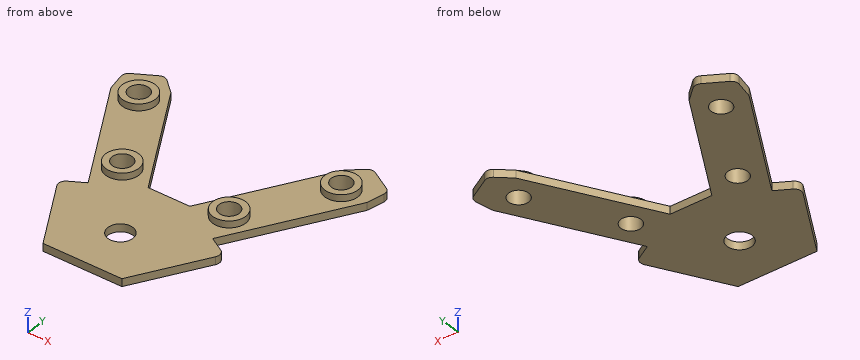
```python
from build123d import *

# Parameters (mm, degrees)
SKETCH1_R             = 2.6
BOSS_EXTRUDE1_DEPTH   = 1.6
SKETCH2_R             = 3.45
BOSS_EXTRUDE2_DEPTH   = 1.4
M5X0_8_TAPPED_HOLE1_D = 4.2


with BuildPart() as part:
    # Sketch1 → Boss-Extrude1 (new body)
    with BuildSketch(Plane.XY):
        with BuildLine():
            Line((-4.364768035, 13.06), (4.364768035, 13.06))
            Line((4.364768035, 13.06), (18.114768035, 36.875698604))
            Line((18.114768035, 36.875698604), (20.854894903, 39.305509792))
            ThreePointArc((20.854894903, 39.305509792), (21.698970531, 39.675572625), (22.600099833, 39.482243506))
            Line((22.600099833, 39.482243506), (26.789690275, 37.063382336))
            ThreePointArc((26.789690275, 37.063382336), (27.407682855, 36.379646028), (27.509236854, 35.463623675))
            Line((27.509236854, 35.463623675), (26.775022073, 31.875698604))
            Line((26.775022073, 31.875698604), (13.025022073, 8.06))
            Line((13.025022073, 8.06), (16.056110986, 6.31))
            ThreePointArc((16.056110986, 6.31), (16.754999726, 5.399190462), (16.605149092, 4.260961894))
            Line((16.605149092, 4.260961894), (8.250335347, -10.21))
            Line((8.250335347, -10.21), (-8.250335347, -10.21))
            Line((-8.250335347, -10.21), (-16.605149092, 4.260961894))
            ThreePointArc((-16.605149092, 4.260961894), (-16.754999726, 5.399190462), (-16.056110986, 6.31))
            Line((-16.056110986, 6.31), (-13.025022073, 8.06))
            Line((-13.025022073, 8.06), (-26.775022073, 31.875698604))
            Line((-26.775022073, 31.875698604), (-27.509236854, 35.463623675))
            ThreePointArc((-27.509236854, 35.463623675), (-27.407682855, 36.379646028), (-26.789690275, 37.063382336))
            Line((-26.789690275, 37.063382336), (-22.600099833, 39.482243506))
            ThreePointArc((-22.600099833, 39.482243506), (-21.698970531, 39.675572625), (-20.854894903, 39.305509792))
            Line((-20.854894903, 39.305509792), (-18.114768035, 36.875698604))
            Line((-18.114768035, 36.875698604), (-4.364768035, 13.06))
        make_face()
        Circle(SKETCH1_R, mode=Mode.SUBTRACT)
    extrude(amount=BOSS_EXTRUDE1_DEPTH)

    # Sketch2 → Boss-Extrude2 (add)
    with BuildSketch(Plane.XY.offset(1.6)):
        with Locations((21.178557159, 32.18233703)):
            Circle(SKETCH2_R)
        with Locations((11.178557159, 14.861828954)):
            Circle(SKETCH2_R)
        with Locations((-11.178557159, 14.861828954)):
            Circle(SKETCH2_R)
        with Locations((-21.178557159, 32.18233703)):
            Circle(SKETCH2_R)
    extrude(amount=BOSS_EXTRUDE2_DEPTH)

    # M5x0.8 Tapped Hole1 (through all)
    with Locations(Plane.XY.offset(3)):
        with Locations((21.178557159, 32.18233703), (11.178557159, 14.861828954), (-11.178557159, 14.861828954), (-21.178557159, 32.18233703)):
            Hole(M5X0_8_TAPPED_HOLE1_D / 2)


solid = part.part
```
Input: part model. Units: mm. Frame: model coordinates. Give positions to 0.01 mm unless a question says otherwise; leave off trailing zeros. Order: outer loops, then holes, each group sorted by start corner. A loop starts at its lowest first (then second) coordinate and runs counter-clockwise, first axis right, second up. Notation, with made-up numbers: M 25,29.25 L 50,29.25 A20 cw 50,67.25 Z; hole C -6.75,88 d10. An arc over 180 degrees is marked long. Return JSON: item names as keys, results as strings.
1) Section query D-D on x = 11. Output: boundary loops of the cut face in (y, z).
Taken from the geometry:
{"outline": "M -5.45,0 L 12.77,0 L 12.77,3 L 11.42,3 L 11.42,1.6 L -5.45,1.6 Z; M 16.95,0 L 24.55,0 L 24.55,1.6 L 18.31,1.6 L 18.31,3 L 16.95,3 Z"}
2) Contact query for flat-ended pins moving along their axis: pin 1 (5.5 mm diameter, centred on x = -11.18, y = 14.86, fed in from -Z); pin 2 (1.5 mm diameter, centred on y = 22, z = 1.5, fed in from -X); pin 3 (1.3 mm diameter, centred on x = -1, z = 0.5, fed in from +Y); pin 4 (1 mm diameter, centred on y = 32, z = 0.5, fed in from +X). Output: stop coordinate, or through.
Taken from the geometry:
{"pin 1": "stops at z = 0", "pin 2": "stops at x = -21.51", "pin 3": "stops at y = 13.06", "pin 4": "stops at x = 26.9"}
3) Section query B-B on y = 28. Output: boundary loops of the cut face in (x, z).
Taken from the geometry:
{"outline": "M -24.54,0 L -12.99,0 L -12.99,1.6 L -24.54,1.6 Z; M 12.99,0 L 24.54,0 L 24.54,1.6 L 12.99,1.6 Z"}
4) Section query A-A on x = 0. Output: boundary loops of the cut face in (y, z), and give its area (3 significant figures).
Taken from the geometry:
{"outline": "M -10.21,0 L -2.6,0 L -2.6,1.6 L -10.21,1.6 Z; M 2.6,0 L 13.06,0 L 13.06,1.6 L 2.6,1.6 Z", "area": "28.9 mm2"}
5) Section query C-C on z = 2.2. Output: boundary loops of the cut face in (x, y), and give its area (3 significant figures).
Taken from the geometry:
{"outline": "C -21.18,32.18 d6.9; C -11.18,14.86 d6.9; C 11.18,14.86 d6.9; C 21.18,32.18 d6.9; hole C -21.18,32.18 d4.2; hole C -11.18,14.86 d4.2; hole C 11.18,14.86 d4.2; hole C 21.18,32.18 d4.2", "area": "94.2 mm2"}
6) Line query: L1, parallel to X at y = 13, z = 1.25; L2, parallel to X at y = 30.5, z = 2.95; L3, parallel to Y at x = 0, z = 0.8. Output: solid intervals per line, ascending. Write a range as [from, to].
Taken from the geometry:
{"L1": "x = [-15.88, -12.15], [-10.21, 10.21], [12.15, 15.88]", "L2": "x = [-24.19, -22.44], [-19.92, -18.17], [18.17, 19.92], [22.44, 24.19]", "L3": "y = [-10.21, -2.6], [2.6, 13.06]"}
